The model under review builds one solid part; all positions refer to its coordinate system, in mm. Face numbers are marked on the shaded views. A direction names the side the tool comes from. Round coordinates to 2 decimals unless told otherwise and drop trailing zeros. Order: outer loops, then holes, each group sorted by start corner. A loop starts at its lowest first (then second) coordinate and runs counter-clockwise, first axis right, second up. Notation, with made-up numbers: M 5.5,-28.75 L 30.5,-28.75 A25 ccw 30.5,3.25 Z; hole C -38.75,46.5 d1. An arc over 180 degrees is marked long. Use a Markdown table: item, result. Add a question column.
1. For the marked faces 1, 2 and 3, list the 3-axis set-ups (+Z, -Z, +X, -X, +Y, -Y) from which the entire face can be reached by the end or side of a thin tool; tool diameter is ignored.
2. Insertion check: P1, Ø3, axis at y = 39.5, z = -12, coming from the +X side. The pin has a flat end and moves straight along its axis. Give the tip position at first contact, or say it passes through.
3. Consider section D-D on y = 51.5. State the section outline as (x, z) points (3 decimals).
4. To check wall thickness, follow probe 1 along Y at (x, z) = (26.5, -13.2) (3 decimals); probe 2 along X at (y, z) = (54.5, -14.25); probe 3 along Y at (x, z) = (38.75, -13.2) (3 decimals). State the ranges of each line that lie inside material, in increasing order.
5. Consider section C-C on x = 31. State the section outline as (y, z) points (3 decimals).
6. Consider section B-B on z = -14.5. State the section outline as (x, y) points (1 decimal), then the cut area to 3 significant figures.
7. Consider section A-A on y = 73.72. State the section outline as (x, z) points (3 decimals), then the cut area to 3 significant figures.
from build123d import *

# Parameters (mm, degrees)
SKETCH2_R                = 7.5
BOSS_EXTRUDE1_DEPTH      = 3.175
BOSS_EXTRUDE1_DEPTH_BACK = 3.175
CUT_EXTRUDE1_REACH       = 27
SKETCH3_R                = 2.325


with BuildPart() as part:
    # Sketch2 → Boss-Extrude1 (new body, two sides)
    with BuildSketch(Plane(origin=(0, 0, -13.2), x_dir=(-1, 0, 0), z_dir=(0, 0, -1))) as boss_extrude1_sk:
        with BuildLine():
            Line((-19.1, 36.72), (-44.1, 36.72))
            Line((-44.1, 36.72), (-44.1, 46.72))
            Line((-44.1, 46.72), (-49.39334567, 46.72))
            ThreePointArc((-49.39334567, 46.72), (-50.77714312, 58.387484646), (-44.1, 68.055))
            Line((-44.1, 68.055), (-44.1, 79.385))
            Line((-44.1, 79.385), (-19.1, 79.385))
            Line((-19.1, 79.385), (-19.1, 36.72))
        make_face()
        with Locations((-34.645, 54.385)):
            Circle(SKETCH2_R, mode=Mode.SUBTRACT)
    extrude(amount=BOSS_EXTRUDE1_DEPTH)
    extrude(boss_extrude1_sk.sketch, amount=-BOSS_EXTRUDE1_DEPTH_BACK)

    # Sketch3 → Cut-Extrude1 (cut, up to next)
    with BuildSketch(Plane(origin=(44.1, 0, 0), x_dir=(0, 0, -1), z_dir=(1, 0, 0)), mode=Mode.PRIVATE) as cut_extrude1_sk1:
        with Locations((13.2, 41.72)):
            Circle(SKETCH3_R)
    cut_extrude1_tool1 = extrude(cut_extrude1_sk1.sketch, amount=-CUT_EXTRUDE1_REACH, mode=Mode.PRIVATE) & part.part
    add(cut_extrude1_tool1.solids().sort_by_distance((44.1, 41.72, -13.2))[0], mode=Mode.SUBTRACT)
    # Sketch3 → Cut-Extrude1 (cut, up to next)
    with BuildSketch(Plane(origin=(44.1, 0, 0), x_dir=(0, 0, -1), z_dir=(1, 0, 0)), mode=Mode.PRIVATE) as cut_extrude1_sk2:
        with Locations((13.2, 73.72)):
            Circle(SKETCH3_R)
    cut_extrude1_tool2 = extrude(cut_extrude1_sk2.sketch, amount=-CUT_EXTRUDE1_REACH, mode=Mode.PRIVATE) & part.part
    add(cut_extrude1_tool2.solids().sort_by_distance((44.1, 73.72, -13.2))[0], mode=Mode.SUBTRACT)


solid = part.part
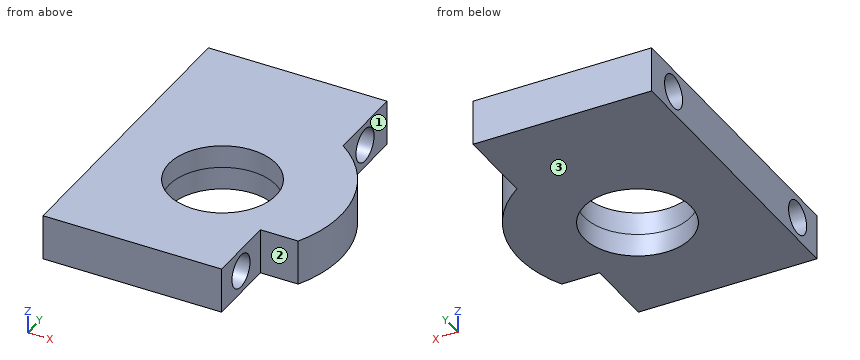
Answer block:
| question | item | result |
|---|---|---|
| 1 | face 1 | +Z, -Z, +X, +Y |
| 1 | face 2 | +Z, -Z, +X, -Y |
| 1 | face 3 | -Z, +X, -X, +Y, -Y |
| 2 | P1 | x = 44.1 |
| 3 | outline | M 19.1,-16.375 L 27.722,-16.375 L 27.722,-10.025 L 19.1,-10.025 Z; M 41.568,-16.375 L 51.014,-16.375 L 51.014,-10.025 L 41.568,-10.025 Z |
| 4 | probe 1 | 36.72 to 39.395, 44.045 to 71.395, 76.045 to 79.385 |
| 4 | probe 2 | 19.1 to 27.15, 42.14 to 51.27 |
| 4 | probe 3 | 36.72 to 39.395, 44.045 to 48.108, 60.662 to 71.395, 76.045 to 79.385 |
| 5 | outline | M 36.72,-16.375 L 47.83,-16.375 L 47.83,-10.025 L 36.72,-10.025 Z; M 60.94,-16.375 L 79.385,-16.375 L 79.385,-10.025 L 60.94,-10.025 Z; hole C 41.72,-13.2 d4.65; hole C 73.72,-13.2 d4.65 |
| 6 | outline | M 19.1,36.7 L 44.1,36.7 L 44.1,39.8 L 19.1,39.8 Z; M 19.1,43.6 L 44.1,43.6 L 44.1,46.7 L 49.4,46.7 A16.6 ccw 44.1,68.1 L 44.1,71.8 L 19.1,71.8 Z; M 19.1,75.6 L 44.1,75.6 L 44.1,79.4 L 19.1,79.4 Z; hole C 34.6,54.4 d15 |
| 6 | area | 816 mm^2 |
| 7 | outline | M 19.1,-16.375 L 44.1,-16.375 L 44.1,-15.525 L 19.1,-15.525 Z; M 19.1,-10.875 L 44.1,-10.875 L 44.1,-10.025 L 19.1,-10.025 Z |
| 7 | area | 42.5 mm^2 |
